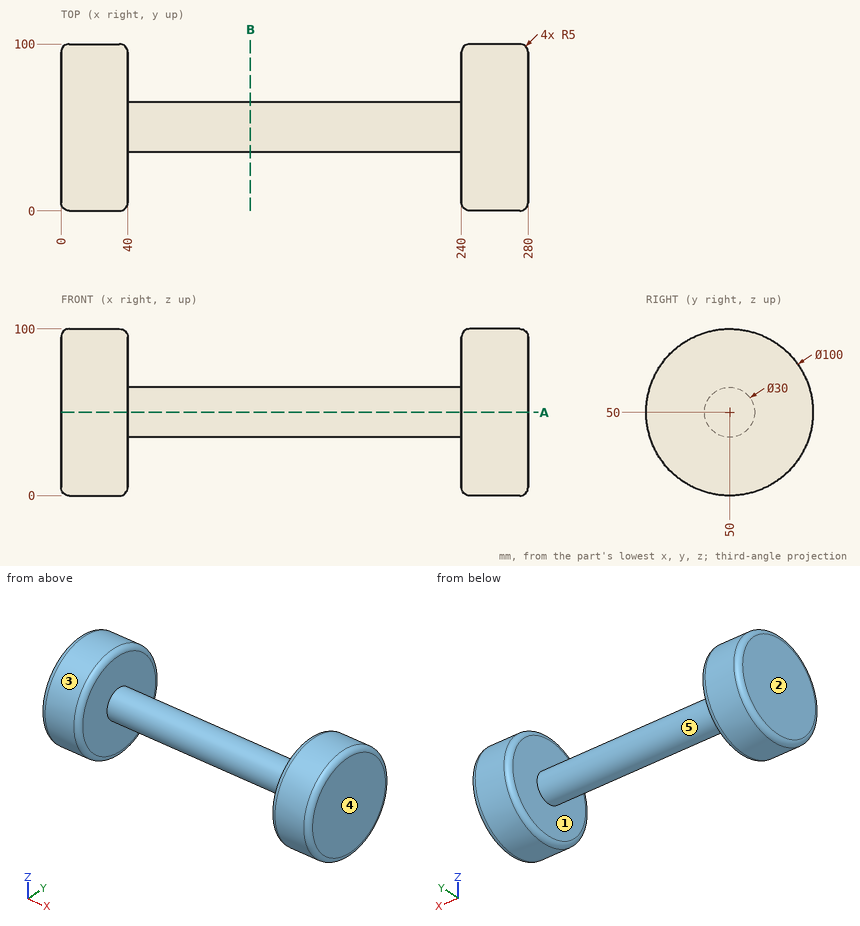
Source: three-view drawing plus pictorial views. Frame: mm from the lowest corner of the part. A direction names the side the tool comes from. Give positions to 0.01 mm unless a question says otherwise; leave off trailing zeros. Write each loop counter-clockwise with the first axis right and the second up, starting at its lowest first coordinate (ties: lowest second). Pieces come first, ordered by that corner, then holes. Notation, with made-up numbers: (-27, -17) -> (18, -17) arc R24 ccw to (18, 20) -> close; hole circle Ø11 at (30.5, 37). An arc over 180 degrees is marked (long way). Write item = value, one per line.
Q1. Reachability of the marked faces 4 and 5 from +Z, -Z, +X, -X, +Y, -Y: full face, straight path, thin tool, end or side. Return the list, or none.
Here are the results:
face_4 = +Z, -Z, +X, +Y, -Y
face_5 = none
Q2. First-contact query: pin 1 (5 mm diameter, centred on x = 84, y = 40.5, fed in from +Z); pin 2 (8 mm diameter, centred on x = 232.5, y = 85, fed in from +Z); pin 3 (2 mm diameter, centred on x = 42, z = 46, fed in from -Y). Flat tips, straight axial feed; report the tip coordinate or a pass-through.
Here are the results:
pin_1 = 63.27
pin_2 = through
pin_3 = 35.3
Q3. Line query: line 1 (X direction, y = 59, z = 78.5); line 2 (X direction, y = 81, z = 88); line 3 (Y direction, x = 27, z = 49.5). Output: solid intervals per line, ascending. Write a range as from..to.
Here are the results:
line_1 = 0..40, 240..280
line_2 = 2.06..37.94, 242.06..277.94
line_3 = 0..100
Q4. Cut plane A-A on z = 50. Return loops of the section in (x, y), then the cut area to 3 significant figures.
Here are the results:
outline = (0, 5) arc R5 ccw to (5, 0) -> (35, 0) arc R5 ccw to (40, 5) -> (40, 35) -> (240, 35) -> (240, 5) arc R5 ccw to (245, 0) -> (275, 0) arc R5 ccw to (280, 5) -> (280, 95) arc R5 ccw to (275, 100) -> (245, 100) arc R5 ccw to (240, 95) -> (240, 65) -> (40, 65) -> (40, 95) arc R5 ccw to (35, 100) -> (5, 100) arc R5 ccw to (0, 95) -> close
area = 14,000 mm²
Q5. Mould query, pull axis X, two halves, no side actions, for the marked faces 1, 2 and 3. Classes: +X half, -X half, draft (parallel to the pull), parting line (faces both ways), or undercut.
Here are the results:
face_1 = undercut
face_2 = -X half
face_3 = draft
Q6. Cut plane B-B on x = 113.5. Return loops of the section in (y, z), then the cut area to 3 significant figures.
Here are the results:
outline = circle Ø30 at (50, 50)
area = 707 mm²
